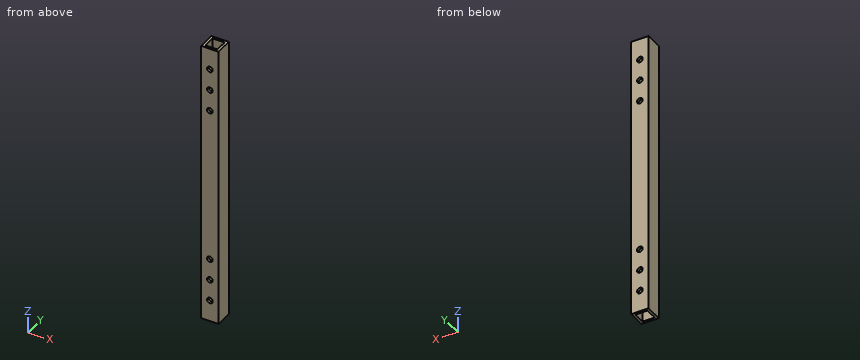
```python
from build123d import *

# Parameters (mm, degrees)
SKETCH_1_W          = 10
SKETCH_1_H          = 10
SKETCH_1_W_2        = 7
SKETCH_1_H_2        = 7
EXTRUDE_1_DEPTH     = 165
SKETCH_2_R          = 1.65
CUT_EXTRUDE_1_DEPTH = 166.378354085


with BuildPart() as part:
    # 草图1 → 凸台-拉伸1 (new body)
    with BuildSketch(Plane.XY):
        Rectangle(SKETCH_1_W, SKETCH_1_H)
        Rectangle(SKETCH_1_W_2, SKETCH_1_H_2, mode=Mode.SUBTRACT)
    extrude(amount=EXTRUDE_1_DEPTH)

    # 草图2 → 切除-拉伸1 (cut, through all)
    with BuildSketch(Plane(origin=(0, 5, 0), x_dir=(1, 0, 0), z_dir=(0, 1, 0))):
        with Locations(Location((0, -12.5, 0), (0, 0, 270))):
            Circle(SKETCH_2_R)
        with Locations(Location((0, -25, 0), (0, 0, 270))):
            Circle(SKETCH_2_R)
        with Locations(Location((0, -37.5, 0), (0, 0, 270))):
            Circle(SKETCH_2_R)
        with Locations(Location((0, -127.5, 0), (0, 0, 270))):
            Circle(SKETCH_2_R)
        with Locations(Location((0, -140, 0), (0, 0, 270))):
            Circle(SKETCH_2_R)
        with Locations(Location((0, -152.5, 0), (0, 0, 270))):
            Circle(SKETCH_2_R)
    extrude(amount=-CUT_EXTRUDE_1_DEPTH, mode=Mode.SUBTRACT)


solid = part.part
```
Work out the finished part from the listing and answer in its coordinate system (mm). Coordinates: 2 decimals unless noted, no trailing zeros. Loops run counter-clockwise (first coordinate to the right, second up) from the corner with the lowest first, then second, coordinate; pieces in that order, holes last. Notation, with made-up numbers: M 50,-30.5 L 87,-30.5 A18 ccw 87,-11.5 Z; hole C -37.5,32 d9. An arc over 180 degrees is marked long. Use CSV: the item, a comma, the result in double quotes. Start each with the question number.
(1) Find section B-B, the plane y = -0.75. Give the vertices of the cut face in (x, z), then the cut area to 3 significant figures.
(2) Find section A-A, the plane z = 152.5. Give the vertices of the cut face in (x, y).
(3) Given pin 1 Ø2.5 at (x, z) = (0, 25) entering from +Y, flat-ended and moving along its own axis, determine where the tip first touches the part or whether it passes through.
(4) Consider line 1 (X direction, y = 0, z = 117); line 2 (X direction, y = -4.35, z = 37.5). Determine where each line is inside the solid, lowest interval first.
(5) Find section C-C, the plane z = 123. Give the vertices of the cut face in (x, y).
(6) Find section D-D, the plane x = 0. State how many separate pieces and enclosed holes the cut face has, then the cut area to 3 significant figures.
Recorded:
1,outline,"M -5,0 L -3.5,0 L -3.5,165 L -5,165 Z; M 3.5,0 L 5,0 L 5,165 L 3.5,165 Z"
1,area,"495 mm^2"
2,outline,"M -5,-5 L -1.65,-5 L -1.65,-3.5 L -3.5,-3.5 L -3.5,3.5 L -1.65,3.5 L -1.65,5 L -5,5 Z; M 1.65,-5 L 5,-5 L 5,5 L 1.65,5 L 1.65,3.5 L 3.5,3.5 L 3.5,-3.5 L 1.65,-3.5 Z"
3,pin 1,"passes through"
4,line 1,"x = -5 to -3.5, 3.5 to 5"
4,line 2,"x = -5 to -1.65, 1.65 to 5"
5,outline,"M -5,-5 L 5,-5 L 5,5 L -5,5 Z; hole M -3.5,-3.5 L 3.5,-3.5 L 3.5,3.5 L -3.5,3.5 Z"
6,separate pieces,"14"
6,enclosed holes,"0"
6,area,"436 mm^2"
